Geometry: final body of the model. Coordinates: model frame, mm. Face numbers are marked on the shaded views. A direction names the side the tool comes from. Give positions to 0.01 mm unless a question says otherwise; leave off trailing zeros. Write each loop counter-clockwise with the first axis right and the second up, starting at its lowest first coordinate (ties: lowest second). Pieces come first, ordered by that corner, then holes. Notation, with made-up numbers: M -36,76 L 5,76 A24 ccw 5,89 Z; hole C 34.5,36.25 d6. An arc over 180 degrees is marked long. Use one line per item in the form item = value. Start each with the question number.
Item 1: Section query D-D on y = 50. Return loops of the section in (x, z).
Item 2: Section query B-B on z = 7.75. Return loops of the section in (x, y), then the cut area to 3 significant figures.
Item 3: Pull-direction query (X, two-part tool) for the marked faces 1 and 2; classes: released by +X, released by -X, zero draft, split by the parting line, or undercut.
Item 4: Access query for the marked faces 3 and 4. Directions: +Z, -Z, +X, -X, +Y, -Y. A direction counts if a zero-diameter tool reaches every point of the face in a straight line with its end or side. Return the directions, or none.
Item 5: Section query C-C on x = 75. Return loops of the section in (y, z).
Item 6: Contact query for flat-ended pins moving along their axis: P1, Ø22.5, axis at x = -70.71, y = 70.71, coming from the -Z side; P2, Ø7, axis at x = -94, y = 0.5, coming from the -Z side. Output: stop coordinate, or through.
Item 7: Section query A-A on x = 0. Return loops of the section in (y, z).
Item 8: Material intervals for line 1 along X through (y, z) = (0, 2.6); line 2 along Y through (x, z) = (0, 1.15); line 3 along X through (y, z) = (70.5, 8.75), sorted ascending. Write a range as from..to.
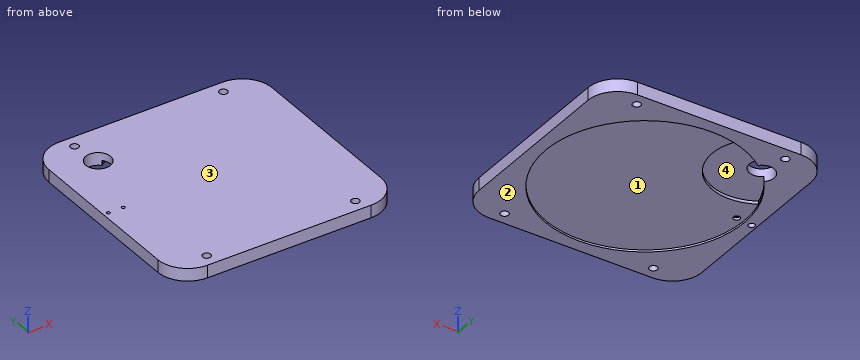
Autodesk Inventor part; units mm, degrees
ref_plane "YZ Plane" through (0, 0, 0) normal (1, 0, 0) x (0, 1, 0)
ref_plane "XZ Plane" through (0, 0, 0) normal (0, 1, 0) x (-1, 0, 0)
ref_plane "XY Plane" through (0, 0, 0) normal (0, 0, 1) x (1, 0, 0)
sketch "Sketch1" plane through (0, 0, 0) normal (0, 0, 1) x (1, 0, 0)
  circle A0 centre (0, 0) radius 100 construction
  line L0 (112.5, 0) -> (112.5, 112.5)
  line L1 (112.5, 112.5) -> (-112.5, 112.5)
  line L2 (-112.5, 112.5) -> (-112.5, -112.5)
  line L3 (-112.5, -112.5) -> (112.5, -112.5)
  line L4 (112.5, -112.5) -> (112.5, 0)
  circle A1 centre (-75, -100) radius 4.05
  circle A2 centre (75, -100) radius 4.05
  line L5 (75, -100) -> (-75, -100) construction
  line L6 (-75, -100) -> (-75, 100) construction
  line L7 (-75, 100) -> (75, 100) construction
  line L8 (75, 100) -> (75, -100) construction
  circle A3 centre (-75, 100) radius 4.05
  circle A4 centre (75, 100) radius 4.05
  point P0 (0, 112.5)
  point P1 (75, 0)
  dimension "d0" = 200
  dimension "d2" = 225
  dimension "d3" = 225
  dimension "d4" = 150
  dimension "d5" = 37.5
  dimension "d6" = 12.5
  dimension "d7" = 8.1
extrude "Extrusion1" add sketch "Sketch1" along normal blind 12.7
fillet "Fillet1" radius 30 4 edges at (-112.5, -112.5, 6.35) (-112.5, 112.5, 6.35) (112.5, -112.5, 6.35) (112.5, 112.5, 6.35)
sketch "Sketch2" plane through (0, 0, 0) normal (0, 0, -1) x (-1, 0, 0)
  circle A0 centre (0, 0) radius 100
  dimension "d14" = 200
extrude "Extrusion2" cut sketch "Sketch2" against normal blind 2
sketch "Sketch4" plane through (0, 0, 0) normal (0, 0, -1) x (-1, 0, 0)
  circle A0 centre (92.5, 0) radius 1.55
  circle A1 centre (107.5, 0) radius 1.55
  circle A2 centre (0, 0) radius 100
  line L0 (112.5, 82.5) -> (112.5, -82.5)
  dimension "d44" = 15
  dimension "d45" = 0
  dimension "d46" = 5
  dimension "d47" = 3.1
hole "Hole1" at (-92.5, 0, 0) at (-107.5, 0, 0) direction (0, 0, 1) diameter 3.4 end through all counterbore diameter 6.5 counterbore depth 4.5
sketch "Sketch5" plane through (0, 0, 2) normal (0, 0, -1) x (-1, 0, 0)
  circle A0 centre (0, 0) radius 100
  circle A1 centre (70.7107, 70.7107) radius 12.5
  line L0 (0, 0) -> (70.7107, 70.7107) construction
  line L1 (82.5, -112.5) -> (-82.5, -112.5) construction
  dimension "d32" = 25
  dimension "d35" = 45
extrude "Extrusion4" cut sketch "Sketch5" along normal through all both and the other way through all contours A1 A0 | A0 A1 picked at (68.0843, 67.4022) picked at (73.7867, 73.4347)
sketch "Sketch6" plane through (0, 0, 2) normal (0, 0, -1) x (-1, 0, 0)
  arc A0 (61.3367, 78.9798) -> (78.9798, 61.3367) centre (70.7107, 70.7107) ccw
  arc A1 (61.3367, 78.9798) -> (78.9798, 61.3367) centre (0, 0) ccw
  arc A2 (27.6392, 96.1045) -> (96.1045, 27.6392) centre (70.7107, 70.7107) ccw
  dimension "d39" = 50
extrude "Extrusion5" cut sketch "Sketch6" against normal blind 3 contours A0 A1 A2
properties part number "board"
Answer sheet:
q1.outline = M -112.5,0 L -86.6,0 L -86.6,5 L -25.2,5 L -25.2,2 L 86.6,2 L 86.6,0 L 112.5,0 L 112.5,12.7 L -112.5,12.7 Z
q2.outline = M -112.5,-82.5 A30 ccw -82.5,-112.5 L 82.5,-112.5 A30 ccw 112.5,-82.5 L 112.5,82.5 A30 ccw 82.5,112.5 L -82.5,112.5 A30 ccw -112.5,82.5 Z; hole C -107.5,0 d3.4; hole C -92.5,0 d3.4; hole C -70.71,70.71 d25; hole C -75,-100 d8.1; hole C -75,100 d8.1; hole C 75,-100 d8.1; hole C 75,100 d8.1
q2.area = 49,100 mm2
q3.face_1 = undercut
q3.face_2 = zero draft
q4.face_3 = +Z, +X, -X, +Y, -Y
q4.face_4 = -Z
q5.outline = M -112.5,0 L -104.05,0 L -104.05,12.7 L -112.5,12.7 Z; M -95.95,0 L -66.14,0 L -66.14,2 L 66.14,2 L 66.14,0 L 95.95,0 L 95.95,12.7 L -95.95,12.7 Z; M 104.05,0 L 112.5,0 L 112.5,12.7 L 104.05,12.7 Z
q6.P1 = through
q6.P2 = 2
q7.outline = M -112.5,0 L -100,0 L -100,2 L 100,2 L 100,0 L 112.5,0 L 112.5,12.7 L -112.5,12.7 Z
q8.line_1 = -112.5..-110.75, -104.25..-95.75, -89.25..112.5
q8.line_2 = -112.5..-100, 100..112.5
q8.line_3 = -112.5..-83.21, -58.21..112.5
